```python
from build123d import *

# Parameters (mm, degrees)
CYLINDER010_R     = 3.5
CYLINDER010_DEPTH = 25
CYLINDER006_R     = 3.5
CYLINDER006_DEPTH = 25
BOX_W             = 19
BOX_H             = 4
BOX_DEPTH         = 100
CYLINDER001_R     = 45
CYLINDER001_DEPTH = 100
CYLINDER_R        = 42.5
CYLINDER_DEPTH    = 100
FILLET_R          = 1
FILLET001_R       = 1


with BuildPart() as cylindre010:
    # Cylinder010 → Cylinder010 (new body)
    with BuildSketch(Plane(origin=(18, -33, -12.5), x_dir=(1, 0, 0), z_dir=(0, 0, 1))):
        Circle(CYLINDER010_R)
    extrude(amount=CYLINDER010_DEPTH)


with BuildPart() as cylindre006:
    # Cylinder006 → Cylinder006 (new body)
    with BuildSketch(Plane(origin=(-18, -33, -12.5), x_dir=(1, 0, 0), z_dir=(0, 0, 1))):
        Circle(CYLINDER006_R)
    extrude(amount=CYLINDER006_DEPTH)


with BuildPart() as cube:
    # Box → Box (new body)
    with BuildSketch(Plane(origin=(-9.5, -39, 0), x_dir=(1, 0, 0), z_dir=(0, 0, 1))):
        with Locations((9.5, 2)):
            Rectangle(BOX_W, BOX_H)
    extrude(amount=BOX_DEPTH)


with BuildPart() as cylindre001:
    # Cylinder001 → Cylinder001 (new body)
    with BuildSketch(Plane(origin=(0, 13, 0), x_dir=(1, 0, 0), z_dir=(0, 0, 1))):
        Circle(CYLINDER001_R)
    extrude(amount=CYLINDER001_DEPTH)


with BuildPart() as cut009:
    # Cylinder → Cylinder (new body)
    with BuildSketch(Plane.XY):
        Circle(CYLINDER_R)
    extrude(amount=CYLINDER_DEPTH)

    # Cut: cut Cylindre001
    add(cylindre001.part, mode=Mode.SUBTRACT)

    # Fillet
    fillet_edges = [cut009.edges().sort_by_distance(p)[0] for p in [
        (-42.456904, -1.913462, 50),
    ]]
    fillet(fillet_edges, radius=FILLET_R)

    # Fillet001
    fillet001_edges = [cut009.edges().sort_by_distance(p)[0] for p in [
        (42.456904, -1.913462, 50),
    ]]
    fillet(fillet001_edges, radius=FILLET001_R)

    # Cut001: cut Cube
    add(cube.part, mode=Mode.SUBTRACT)

    # Cut006: cut Cylindre006
    add(cylindre006.part, mode=Mode.SUBTRACT)

    # Cut009: cut Cylindre010
    add(cylindre010.part, mode=Mode.SUBTRACT)


solid = cut009.part
```
Design review of the part built by this model. Coordinates are the model's own, in mm. A direction names the side the tool comes from. Coordinates: 2 decimals unless noted, no trailing zeros. Write each loop counter-clockwise with the first axis right and the second up, starting at its lowest first coordinate (ties: lowest second). Pieces come first, ordered by that corner, then holes.
1) Add section C-C (x = 18). Write out the cut boundary in (y, z), plus the area to 3 significant figures.
2) Add section B-B (x = 1.5). Write out the cut boundary in (y, z) (3 decimals), plus the area to 3 significant figures.
3) Add section A-A (y = -16). Write out the cut boundary in (x, z).
4) Insertion check: pin 1 (5.5 mm diameter, centred on x = 2.5, z = 46.5, fed in from -Y); pin 2 (7.5 mm diameter, centred on x = 19, y = -33.5, fed in from -Z); pin 3 (8 mm diameter, centred on y = -22.5, z = 38, fed in from +X); pin 4 (1 mm diameter, centred on y = -34, z = 11, fed in from -X). Each pin has a flat end and moves straight along its axis. Give the tip position at first contact, or say it passes through.
5) Machinability: for faces 4 (the flat face through (-3, -33, 0)), 5 (the flat face through (0, -35, 49)), 6 (the cylindrical face through (17.54, -29.53, 6.16)), which of the approach directions +Z, -Z, +X, -X, +Y, -Y give a long, thin tool a straight path to every point of the face, cutting with its end or side? Answer none if there is none.
6) Mouldability with a two-part tool opening along X and no side actions: class faces 1 (the cylindrical face through (-0.81, -42.492, 49.3)), 2 (the flat face through (3, -33, 100)), 3 (the flat face through (-9.5, -37, 49)) as +X half, -X half, draft (parallel to the pull), parting line (faces both ways), or undercut.
7) To check wall thickness, follow L1, parallel to X at y = -33, z = 5.75; L2, parallel to X at y = -16, z = 68.5; L3, parallel to Y at x = -18, z = 6.5. State the ranges of each line that lie inside material, in increasing order.
8) Add section D-D (x = -16). Write out the cut boundary in (y, z), plus the area to 3 significant figures.
Check result:
1. outline: (-38.5, 0) - (-36.5, 0) - (-36.5, 12.5) - (-29.5, 12.5) - (-29.5, 0) - (-28.24, 0) - (-28.24, 100) - (-38.5, 100) - close
1. area: 938 mm2
2. outline: (-42.474, 0) - (-39, 0) - (-39, 100) - (-42.474, 100) - close; (-35, 0) - (-31.975, 0) - (-31.975, 100) - (-35, 100) - close
2. area: 650 mm2
3. outline: (-39.37, 0) - (-34.41, 0) - (-34.41, 100) - (-39.37, 100) - close; (34.41, 0) - (39.37, 0) - (39.37, 100) - (34.41, 100) - close
4. pin 1: stops at y = -42.5
4. pin 2: stops at z = 0
4. pin 3: stops at x = 38.26
4. pin 4: stops at x = -26.15
5. face 4: -Z, +X, -X, +Y, -Y
5. face 5: +Z, -Z
5. face 6: -Z
6. face 1: parting line
6. face 2: draft
6. face 3: undercut
7. L1: x = -26.78 to -21.5, -14.5 to 14.5, 21.5 to 26.78
7. L2: x = -39.37 to -34.41, 34.41 to 39.37
7. L3: y = -38.5 to -36.5, -29.5 to -28.24
8. outline: (-39.37, 0) - (-35.87, 0) - (-35.87, 12.5) - (-30.13, 12.5) - (-30.13, 0) - (-29.06, 0) - (-29.06, 100) - (-39.37, 100) - close
8. area: 960 mm2
